Model file for the job. Use its own axes, mm. Face numbers are marked on the shaded views. A direction names the side the tool comes from. Coordinates: 2 decimals unless noted, no trailing zeros. Write each loop counter-clockwise with the first axis right and the second up, starting at its lowest first coordinate (ties: lowest second). Pieces come first, ordered by that corner, then holes. Notation, with made-up numbers: M 59,-21.75 L 109,-21.75 A33 cw 109,6.25 Z; hole C 23.25,32 d11. An arc over 180 degrees is marked long. Put each result on its own line as item: value. Start each with the question number.
Q1. Which spindle directions (+Z, -Z, +X, -X, +Y, -Y) get a long thin tool onto all of the face, cutting with end or side? Do the marked faces 5, 6, 7 and 8. Say none if no direction does.
Q2. Drill centre lines: line 1 along Z through (x, y) = (-69.5, 95); line 2 along X through (y, z) = (23, -20); line 3 along Y through (x, z) = (-63.5, -21). Where is each one in solid material? Low to high.
Q3. Cut at D-D (y = 8). Write the cut outline in (x, z), then the cut area to 3 significant figures.
Q4. Cut at B-B (y = 85). Write the cut outline in (x, z), then the cut area to 3 significant figures.
Q5. Drop flat-ended pins along their axis: pin 1 (1.5 mm diameter, centred on y = 64, z = -43, fed in from +X); pin 2 (11 mm diameter, centred on x = -63.5, z = -33.5, fed in from +Y); pin 3 (6 mm diameter, centred on x = -66, y = 94, fed in from -Z). Give the stop position or say it passes through.
Q6. Cut at C-C (z = -43). Write the cut outline in (x, y).
Q7. Cut at A-A (x = -59.5). Write the cut outline in (y, z), then the cut area to 3 significant figures.
Q8. Pull direction X, two halves, no side cores. Call the marked faces 1, 2, 3 and 4: pulls with the +X half, pulls with the -X half, needs draft (parallel to the pull), parting line crosses it, or undercut.
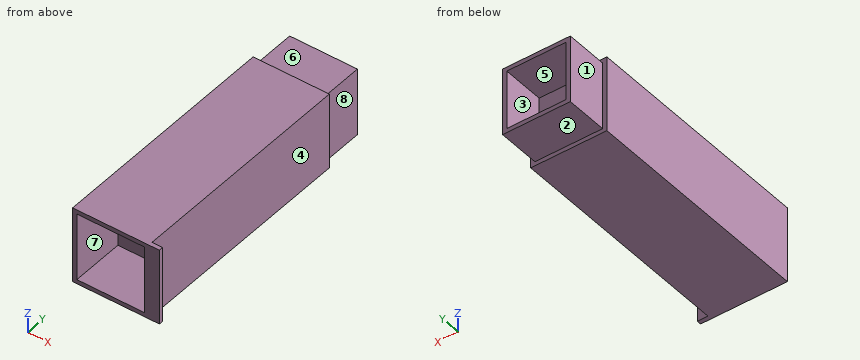
```python
from build123d import *

# Parameters (mm, degrees)
SKETCH1_W           = 36
SKETCH1_H           = 36
SKETCH1_W_2         = 32
SKETCH1_H_2         = 32
BOSS_EXTRUDE1_DEPTH = 76.2
SKETCH2_W           = 36
SKETCH2_H           = 36
BOSS_EXTRUDE2_DEPTH = 5
SKETCH3_W           = 36
SKETCH3_H           = 36
SKETCH3_W_2         = 32
SKETCH3_H_2         = 32
BOSS_EXTRUDE3_DEPTH = 25.4
SKETCH4_W           = 36
SKETCH4_H           = 2
BOSS_EXTRUDE4_DEPTH = 5
SKETCH5_W           = 36
SKETCH5_H           = 36
BOSS_EXTRUDE5_DEPTH = 5
SKETCH6_W           = 32
SKETCH6_H           = 32
SKETCH6_W_2         = 28
SKETCH6_H_2         = 28
BOSS_EXTRUDE6_DEPTH = 20


with BuildPart() as part:
    # Sketch1 → Boss-Extrude1 (new body)
    with BuildSketch(Plane(origin=(0, 0, 0), x_dir=(1, 0, 0), z_dir=(0, 1, 0))):
        with Locations((-61.04447382, 32.009277239)):
            Rectangle(SKETCH1_W, SKETCH1_H)
        with Locations((-61.04447382, 32.009277239)):
            Rectangle(SKETCH1_W_2, SKETCH1_H_2, mode=Mode.SUBTRACT)
    extrude(amount=BOSS_EXTRUDE1_DEPTH)

    # Sketch2 → Boss-Extrude2 (add)
    with BuildSketch(Plane.XZ):
        with Locations((-61.04447382, -32.009277239)):
            Rectangle(SKETCH2_W, SKETCH2_H)
    extrude(amount=BOSS_EXTRUDE2_DEPTH)

    # Sketch3 → Boss-Extrude3 (add)
    with BuildSketch(Plane.XZ.offset(5)):
        with Locations((-61.04447382, -32.009277239)):
            Rectangle(SKETCH3_W, SKETCH3_H)
        with Locations((-61.04447382, -32.009277239)):
            Rectangle(SKETCH3_W_2, SKETCH3_H_2, mode=Mode.SUBTRACT)
    extrude(amount=BOSS_EXTRUDE3_DEPTH)

    # Sketch4 → Boss-Extrude4 (add)
    with BuildSketch(Plane(origin=(-43.04447382, 0, 0), x_dir=(0, 0, -1), z_dir=(1, 0, 0))):
        with Locations((32.009277239, -29.4)):
            Rectangle(SKETCH4_W, SKETCH4_H)
    extrude(amount=BOSS_EXTRUDE4_DEPTH)

    # Sketch5 → Boss-Extrude5 (add)
    with BuildSketch(Plane(origin=(0, 76.2, 0), x_dir=(1, 0, 0), z_dir=(0, 1, 0))):
        with Locations((-61.04447382, 32.009277239)):
            Rectangle(SKETCH5_W, SKETCH5_H)
    extrude(amount=BOSS_EXTRUDE5_DEPTH)

    # Sketch6 → Boss-Extrude6 (add)
    with BuildSketch(Plane(origin=(0, 81.2, 0), x_dir=(1, 0, 0), z_dir=(0, 1, 0))):
        with Locations((-61.04447382, 32.009277239)):
            Rectangle(SKETCH6_W, SKETCH6_H)
        with Locations((-61.04447382, 32.009277239)):
            Rectangle(SKETCH6_W_2, SKETCH6_H_2, mode=Mode.SUBTRACT)
    extrude(amount=BOSS_EXTRUDE6_DEPTH)


solid = part.part
```
Computed values:
1. face 5: +Y
1. face 6: +Z, +X, -X, +Y
1. face 7: -Y
1. face 8: +Z, -Z, +X, +Y
2. line 1: -48.01 to -46.01, -18.01 to -16.01
2. line 2: -79.04 to -77.04, -45.04 to -43.04
2. line 3: -5 to 0, 76.2 to 81.2
3. outline: M -79.04,-50.01 L -43.04,-50.01 L -43.04,-14.01 L -79.04,-14.01 Z; hole M -77.04,-48.01 L -45.04,-48.01 L -45.04,-16.01 L -77.04,-16.01 Z
3. area: 272 mm2
4. outline: M -77.04,-48.01 L -45.04,-48.01 L -45.04,-16.01 L -77.04,-16.01 Z; hole M -75.04,-46.01 L -47.04,-46.01 L -47.04,-18.01 L -75.04,-18.01 Z
4. area: 240 mm2
5. pin 1: x = -43.04
5. pin 2: y = 81.2
5. pin 3: z = -48.01
6. outline: M -79.04,-30.4 L -77.04,-30.4 L -77.04,-5 L -45.04,-5 L -45.04,-30.4 L -38.04,-30.4 L -38.04,-28.4 L -43.04,-28.4 L -43.04,81.2 L -45.04,81.2 L -45.04,101.2 L -47.04,101.2 L -47.04,81.2 L -75.04,81.2 L -75.04,101.2 L -77.04,101.2 L -77.04,81.2 L -79.04,81.2 Z; hole M -77.04,0 L -45.04,0 L -45.04,76.2 L -77.04,76.2 Z
7. outline: M -30.4,-50.01 L 81.2,-50.01 L 81.2,-48.01 L 101.2,-48.01 L 101.2,-46.01 L 81.2,-46.01 L 81.2,-18.01 L 101.2,-18.01 L 101.2,-16.01 L 81.2,-16.01 L 81.2,-14.01 L -30.4,-14.01 L -30.4,-16.01 L -5,-16.01 L -5,-48.01 L -30.4,-48.01 Z; hole M 0,-48.01 L 76.2,-48.01 L 76.2,-16.01 L 0,-16.01 Z
7. area: 846 mm2
8. face 1: pulls with the -X half
8. face 2: needs draft
8. face 3: undercut
8. face 4: pulls with the +X half
